Input: part model. Units: mm. Frame: model coordinates. Face numbers are marked on the shaded views. A direction names the side the tool comes from. Give positions to 0.01 mm unless a question says otherwise; leave off trailing zeros. Order: outer loops, then holes, each group sorted by start corner. A loop starts at its lowest first (then second) coordinate and runs counter-clockwise, first axis right, second up. Notation, with made-up numbers: M -25.75,0.5 L 11.25,0.5 A14 ccw 11.25,19.5 Z; hole C -24,77.25 d10. An arc over 180 degrees is marked long. Use a Markdown table: item, result.
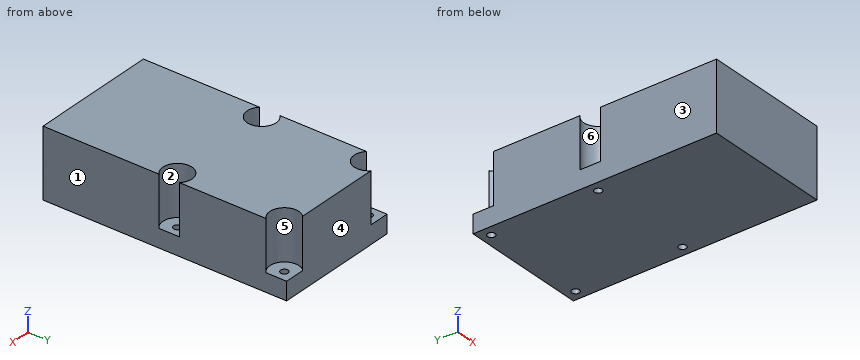
Solid Edge part; units mm, degrees
sketch "Sketch1" plane through (0, 0, 0) normal (0, 0, 1) x (1, 0, 0)
  line L0 (0, 0) -> (56, 0)
  line L1 (56, 0) -> (56, 107)
  line L2 (56, 107) -> (0, 107)
  line L3 (0, 107) -> (0, 0)
extrude "Protrusion1" add sketch "Sketch1" along normal blind 30
sketch "Sketch2" plane through (28, 53.5, 30) normal (0, 0, 1) x (1, 0, 0)
  circle A0 centre (23.5, 49) radius 1.65
  circle A1 centre (-23.5, 2) radius 1.65
  circle A2 centre (23.5, 2) radius 1.65
  circle A3 centre (-23.5, 49) radius 1.65
extrude "ExtrudedCutout_1" cut sketch "Sketch2" against normal blind 30
sketch "Sketch3" plane through (28, 53.5, 30) normal (0, 0, 1) x (1, 0, 0)
  circle A0 centre (23.5, 49) radius 6.364
  circle A1 centre (-23.5, 2) radius 6.365
  circle A2 centre (23.5, 2) radius 6.365
  circle A3 centre (-23.5, 49) radius 6.364
extrude "ExtrudedCutout_2" cut sketch "Sketch3" against normal blind 22
1) Cut plane A-A on y = 102.5. Return loops of the section in (x, z).
Response values:
| item | result |
|---|---|
| outline | M 0,0 L 2.85,0 L 2.85,8 L 0,8 Z; M 6.15,0 L 49.85,0 L 49.85,8 L 45.14,8 L 45.14,30 L 10.86,30 L 10.86,8 L 6.15,8 Z; M 53.15,0 L 56,0 L 56,8 L 53.15,8 Z |
2) First-contact query: pin 1 Ø5.5 at (x, y) = (49.5, 103) entering from +Z; pin 2 Ø3 at (x, y) = (4.5, 102.5) entering from -Z; pin 3 Ø1.5 at (y, z) = (58.5, 25) entering from +X. Flat tips, straight axial feed; report the tip coordinate or a pass-through.
Response values:
| item | result |
|---|---|
| pin 1 | stops at z = 8 |
| pin 2 | passes through |
| pin 3 | stops at x = 46.36 |
3) Cut plane D-D on z = 13. Return loops of the section in (x, y) (3 decimals), and give its area (3 significant figures).
Response values:
| item | result |
|---|---|
| outline | M 0,0 L 56,0 L 56,50.999 A6.365 cw long 56,60.001 L 56,98 A6.364 cw 47,107 L 9,107 A6.364 cw 0,98 L 0,60.001 A6.365 cw long 0,50.999 Z |
| area | 5,550 mm² |
4) Cut plane B-B on x = 51.5. Return loops of the section in (y, z) (3 decimals).
Response values:
| item | result |
|---|---|
| outline | M 0,0 L 53.85,0 L 53.85,8 L 49.135,8 L 49.135,30 L 0,30 Z; M 57.15,0 L 100.85,0 L 100.85,8 L 96.136,8 L 96.136,30 L 61.865,30 L 61.865,8 L 57.15,8 Z; M 104.15,0 L 107,0 L 107,8 L 104.15,8 Z |
5) Material intervals for line 1 (X direction, y = 102.5, z = 2.5); line 2 (Y direction, x = 4.5, z = 5.75); line 3 (Y direction, x = 52, z = 11), sorted ascending. Write a range as from..to.
Response values:
| item | result |
|---|---|
| line 1 | x = 0..2.85, 6.15..49.85, 53.15..56 |
| line 2 | y = 0..53.85, 57.15..100.85, 104.15..107 |
| line 3 | y = 0..49.15, 61.85..96.16 |
6) Cut plane C-C on y = 55.5. Return loops of the section in (x, z) (3 decimals).
Response values:
| item | result |
|---|---|
| outline | M 0,0 L 2.85,0 L 2.85,8 L 0,8 Z; M 6.15,0 L 49.85,0 L 49.85,8 L 45.135,8 L 45.135,30 L 10.865,30 L 10.865,8 L 6.15,8 Z; M 53.15,0 L 56,0 L 56,8 L 53.15,8 Z |
7) Mould query, pull axis Y, two halves, no side actions, for the marked faces 3, 4, 5 and 6. Classes: released by +Y, released by -Y, zero draft, split by the parting line, or undercut.
Response values:
| item | result |
|---|---|
| face 3 | zero draft |
| face 4 | released by +Y |
| face 5 | undercut |
| face 6 | undercut |
8) Reachability of the marked faces 1 and 2 from +Z, -Z, +X, -X, +Y, -Y: full face, straight path, thin tool, end or side. Return the list, or none.
Response values:
| item | result |
|---|---|
| face 1 | +Z, -Z, +X, +Y, -Y |
| face 2 | +Z |
